Build history of the part. All positions in model axes, mm. Face numbers are marked on the shaded views. Round coordinates to 2 decimals unless told otherwise and drop trailing zeros. Write each loop counter-clockwise with the first axis right and the second up, starting at its lowest first coordinate (ties: lowest second). Pieces come first, ordered by that corner, then holes. Notation, with made-up numbers: M 4,17.25 L 36,17.25 A6 cw 36,23.25 Z; hole C 53,19 d3. An arc over 180 degrees is marked long. Write item = value, one per line.
Autodesk Inventor part; units mm, degrees
ref_plane "YZ Plane" through (0, 0, 0) normal (1, 0, 0) x (0, 1, 0)
ref_plane "XZ Plane" through (0, 0, 0) normal (0, 1, 0) x (-1, 0, 0)
ref_plane "XY Plane" through (0, 0, 0) normal (0, 0, 1) x (1, 0, 0)
sketch "Sketch1" plane through (0, 0, 0) normal (1, 0, 0) x (0, 1, 0)
  line L0 (6.5, -3.7528) -> (0, -7.5056)
  line L1 (0, -7.5056) -> (-6.5, -3.7528)
  line L2 (-6.5, -3.7528) -> (-6.5, 3.7528)
  line L3 (-6.5, 3.7528) -> (0, 7.5056)
  line L4 (0, 7.5056) -> (6.5, 3.7528)
  line L5 (6.5, 3.7528) -> (6.5, -3.7528)
  line L6 (0, 10.5078) -> (0, -10.5078)
  circle A0 centre (0, 0) radius 4
  dimension "d0" = 6.5
  dimension "d1" = 8
extrude "Extrusion1" add sketch "Sketch1" along normal blind 6 contours L0 L6 A0 L4 L5 | L1 L2 L3 L6 A0
properties part number "OcM8"
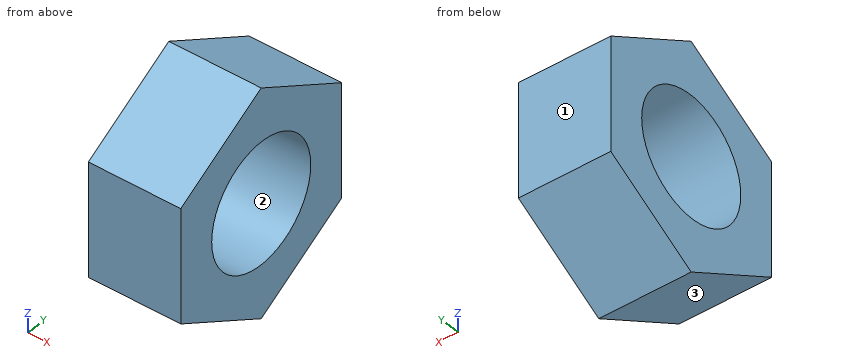
1. Band-saw the part on B-B (x = 3.55). List the corners of the cut face in (y, z).
Responses:
outline = M -6.5,-3.75 L 0,-7.51 L 6.5,-3.75 L 6.5,3.75 L 0,7.51 L -6.5,3.75 Z; hole C 0,0 d8
2. Flat gauge pins, fed straight in: pin 1 (3 mm diameter, centred on x = 2, y = 5, fed in from -Z); pin 2 (3 mm diameter, centred on x = 3, y = -4.5, fed in from +Z); pin 3 (6 mm diameter, centred on y = 0, z = -3.5, fed in from +X). Where does each tip first touch, or does it go through?
Responses:
pin_1 = -5.48
pin_2 = 5.77
pin_3 = 6
3. Band-saw the part on C-C (y = -1.75). List the corners of the cut face in (x, z).
Responses:
outline = M 0,-6.5 L 6,-6.5 L 6,-3.6 L 0,-3.6 Z; M 0,3.6 L 6,3.6 L 6,6.5 L 0,6.5 Z
4. Probe probe 1 along Y at (x, z) = (1.65, 0); probe 2 along Z at (x, y) = (1.1, 1); probe 3 along Y at (x, z) = (2.45, 2.25). List the from-to ranges inside material, lowest first.
Responses:
probe_1 = -6.5 to -4, 4 to 6.5
probe_2 = -6.93 to -3.87, 3.87 to 6.93
probe_3 = -6.5 to -3.31, 3.31 to 6.5
5. Band-saw the part on A-A (z = 0). List the corners of the cut face in (x, y).
Responses:
outline = M 0,-6.5 L 6,-6.5 L 6,-4 L 0,-4 Z; M 0,4 L 6,4 L 6,6.5 L 0,6.5 Z
6. Mould opens along Z. For the marked faces 1, 2 and 3 say: pulls with the +Z half, pulls with the -Z half, needs draft (parallel to the pull), parting line crosses it, or undercut.
Responses:
face_1 = needs draft
face_2 = undercut
face_3 = pulls with the -Z half
7. Band-saw the part on D-D (y = 4.5). List the corners of the cut face in (x, z).
Responses:
outline = M 0,-4.91 L 6,-4.91 L 6,4.91 L 0,4.91 Z
